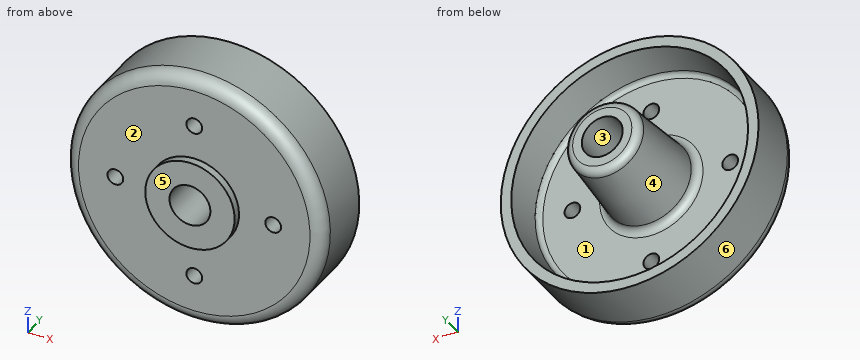
```python
from build123d import *

# Parameters (mm, degrees)
CUT_EXTRUDE2_START = -45
SKETCH6_R          = 3
CUT_EXTRUDE2_DEPTH = 49
CIRPATTERN2_COUNT  = 4


with BuildPart() as part:
    # Sketch3 → Revolve3 (revolve)
    with BuildSketch(Plane.XY, mode=Mode.PRIVATE) as revolve3_sk:
        with BuildLine():
            Line((-11.253050324, 0), (-7.777152082, 0))
            Line((-7.777152082, 0), (-7.777152082, -47))
            Line((-7.777152082, -47), (-17, -47))
            Line((-17, -47), (-17, -44))
            Line((-17, -44), (-44, -44))
            ThreePointArc((-44, -44), (-47.535533906, -42.535533906), (-49, -39))
            Line((-49, -39), (-49, -19))
            Line((-49, -19), (-45, -19))
            Line((-45, -19), (-43.231423008, -32.26432744))
            ThreePointArc((-43.231423008, -32.26432744), (-42.566416469, -33.504768235), (-41.248967207, -34))
            Line((-41.248967207, -34), (-19.668701252, -34))
            ThreePointArc((-19.668701252, -34), (-17.645287665, -33.214903487), (-16.680924046, -31.270531637))
            Line((-16.680924046, -31.270531637), (-16.679706085, -31.256728077))
            Line((-16.679706085, -31.256728077), (-14.242146839, -2.744457398))
            ThreePointArc((-14.242146839, -2.744457398), (-13.282012151, -0.790177857), (-11.253050324, 0))
        make_face()
    revolve(revolve3_sk.sketch.rotate(Axis((0, 0, 0), (0, -1, 0)), 270), axis=Axis((0, 0, 0), (0, -1, 0)))  # turned: the seam where the file's is

    # Sketch6 → Cut-Extrude2 (cut)
    with BuildSketch(Plane.XZ.offset(44).offset(CUT_EXTRUDE2_START)):
        with Locations(Location((0, 30, 0), (0, 0, 270))):  # turned: the seam where the file's is
            Circle(SKETCH6_R)
    cut_extrude2 = extrude(amount=CUT_EXTRUDE2_DEPTH, mode=Mode.SUBTRACT)

    # CirPattern2: Cut-Extrude2 ×4 about axis
    cirpattern2_axis = Axis((0, 0, 0), (0, 1, 0))
    for i in range(1, CIRPATTERN2_COUNT):
        add(cut_extrude2.rotate(cirpattern2_axis, i * 360 / CIRPATTERN2_COUNT), mode=Mode.SUBTRACT)


solid = part.part
```
CAD build for the part. Positions are in the model's coordinates, mm. Face numbers are marked on the shaded views. A direction names the side the tool comes from. Coordinates: 2 decimals unless noted, no trailing zeros. Order: outer loops, then holes, each group sorted by start corner. A loop starts at its lowest first (then second) coordinate and runs counter-clockwise, first axis right, second up. Notation, with made-up numbers: (76.25, 0.5) - (97.25, 0.5) arc R12 cw to (97.25, 19.5) - close; hole circle Ø1 at (-27.75, 17). An arc over 180 degrees is marked (long way). Use a Markdown table: item, result. Add a question column.
(1) Flat gauge pins, fed straight in: pin 1 (9.5 mm diameter, centred on x = -30, z = 0, fed in from +Y); pin 2 (2 mm diameter, centred on x = -2.5, y = -26, fed in from -Z); pin 3 (3 mm diameter, centred on x = 20, y = -29.5, fed in from +Z); pin 4 (14 mm diameter, centred on x = 0, z = 0, fed in from -Y). Where does each tip first touch, or does it go through?
(2) Saw through at A-A (y = -20.5). Give the cut face in (x, z), then the cut area to 3 significant figures.
(3) Saw through at B-B (z = 0). Count the separate pieces of the cut face and the enclosed holes in it, then the cut area to 3 significant figures.
(4) Drill centre lines: line 1 along X through (y, z) = (-33, 10.5); line 2 along X through (y, z) = (-36, 30). Where is each one in solid material? Low to high. Write a range as [from, to].
(5) Pull direction X, two halves, no side cores. Call the marked faces 4, 5 and 6: +X half, -X half, draft (parallel to the pull), parting line (faces both ways), or undercut.
(6) Which spindle directions (+Z, -Z, +X, -X, +Y, -Y) get a long thin tool onto all of the face, cutting with end or side? Do the marked faces 1, 2 and 3. Say none if no direction does.
(7) Saw through at D-D (y = -5.5). Give the cut face in (x, z).
Solved:
| question | item | result |
|---|---|---|
| 1 | pin 1 | stops at y = -34 |
| 1 | pin 2 | stops at z = -48.98 |
| 1 | pin 3 | stops at z = 45.37 |
| 1 | pin 4 | passes through |
| 2 | outline | circle Ø98 at (0, 0); circle Ø31.52 at (0, 0); hole circle Ø89.6 at (0, 0); hole circle Ø15.55 at (0, 0) |
| 2 | area | 1,830 mm² |
| 3 | separate pieces | 4 |
| 3 | enclosed holes | 0 |
| 3 | area | 1,420 mm² |
| 4 | line 1 | x = [-47.86, -41.68], [-13.92, 13.92], [41.68, 47.86] |
| 4 | line 2 | x = [-38.74, -3], [3, 38.74] |
| 5 | face 4 | undercut |
| 5 | face 5 | draft |
| 5 | face 6 | parting line |
| 6 | face 1 | +Y |
| 6 | face 2 | -Y |
| 6 | face 3 | +Y, -Y |
| 7 | outline | circle Ø28.96 at (0, 0); hole circle Ø15.55 at (0, 0) |
